Check sheet for the modelled part. Datum: model origin and axes. Units: mm. Face numbers are marked on the shaded views. A direction names the side the tool comes from. Give positions to 0.01 mm unless a question says otherwise; leave off trailing zeros. Write each loop counter-clockwise with the first axis right and the second up, starting at its lowest first coordinate (ties: lowest second). Pieces come first, ordered by that corner, then holes. Notation, with made-up numbers: M -34,50 L -8,50 A13 cw -8,60 Z; hole C -39,56 d11. An arc over 180 degrees is marked long. Write item = value, one per line. Start each with the question number.
1) Cross-section at A-A, the plane x = 0. Record the cut outline in (y, z).
2) Cross-section at D-D, the plane y = -1.5. Record the cut outline in (x, z), plus the area to 3 significant figures.
3) Access from +Z, -Z, +X, -X, +Y, -Y to the whole of each face (thin tool, end or side, straight path). Record for the marked faces 1 and 2.
4) Mould release check, pull along Z, two halves, no side actions. Record for the marked faces 3, 4 and 5: released by +Z, released by -Z, zero draft, split by the parting line, or undercut.
5) Go/stop test with a flat-tipped pin: pin 1 (1.5 mm diameter, centred on x = 10.5, y = 1.5, fed in from -Z). Record where the tip stops, or that it passes through.
6) Cross-section at B-B, the plane z = 0. Record the cut outline in (x, y), plus the area to 4 significant figures.
7) Cross-section at C-C, the plane y = 3. Record the cut outline in (x, z), plus the area to 3 significant figures.
8) Scan lines: line 1 along Z through (x, y) = (0, 2.5); line 2 along X through (y, z) = (-0.4, 0). Record each from-to range of solid material in increasing order. Write a range as [from, to].
```python
from build123d import *

# Parameters (mm, degrees)
SKETCH_1_R      = 15
SKETCH_1_R_2    = 12.75
EXTRUDE_1_DEPTH = 3.5
SKETCH_2_R      = 17
SKETCH_2_R_2    = 12.75
EXTRUDE_2_DEPTH = 3
CHAMFER_1_SIZE  = 2


with BuildPart() as part:
    # 草图1 → 凸台-拉伸1 (new body)
    with BuildSketch(Plane(origin=(0, 0, 0), x_dir=(1, 0, 0), z_dir=(0, 1, 0))):
        Circle(SKETCH_1_R)
        Circle(SKETCH_1_R_2, mode=Mode.SUBTRACT)
    extrude(amount=EXTRUDE_1_DEPTH)

    # 草图2 → 凸台-拉伸2 (add)
    with BuildSketch(Plane(origin=(0, 0, 0), x_dir=(-1, 0, 0), z_dir=(0, -1, 0))):
        Circle(SKETCH_2_R)
        Circle(SKETCH_2_R_2, mode=Mode.SUBTRACT)
    extrude(amount=EXTRUDE_2_DEPTH)

    # 倒角1
    chamfer_1_edges = [part.edges().sort_by_distance(p)[0] for p in [
        (12.75, -3, 0),
    ]]
    chamfer(chamfer_1_edges, length=CHAMFER_1_SIZE)


solid = part.part
```
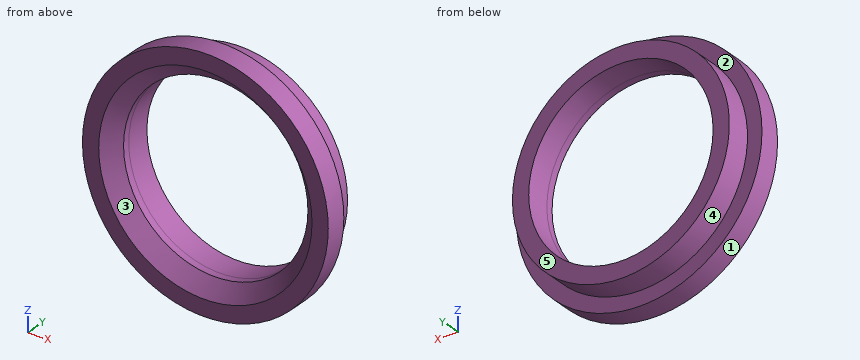
Reply:
q1.outline = M -3,-17 L 0,-17 L 0,-15 L 3.5,-15 L 3.5,-12.75 L -1,-12.75 L -3,-14.75 Z; M -3,14.75 L -1,12.75 L 3.5,12.75 L 3.5,15 L 0,15 L 0,17 L -3,17 Z
q2.outline = C 0,0 d34; hole C 0,0 d26.5
q2.area = 356 mm2
q3.face_1 = +Y, -Y
q3.face_2 = +Y
q4.face_3 = undercut
q4.face_4 = split by the parting line
q4.face_5 = zero draft
q5.pin_1 = -11.4
q6.outline = M -17,-3 L -14.75,-3 L -12.75,-1 L -12.75,3.5 L -15,3.5 L -15,0 L -17,0 Z; M 12.75,-1 L 14.75,-3 L 17,-3 L 17,0 L 15,0 L 15,3.5 L 12.75,3.5 Z
q6.area = 37.25 mm2
q7.outline = C 0,0 d30; hole C 0,0 d25.5
q7.area = 196 mm2
q8.line_1 = [-15, -12.75], [12.75, 15]
q8.line_2 = [-17, -12.75], [12.75, 17]
